from build123d import *

# Parameters (mm, degrees)
SKETCH1_R           = 0.775
BOSS_EXTRUDE1_DEPTH = 18
SKETCH2_R           = 1.5
BOSS_EXTRUDE2_DEPTH = 1
SKETCH3_R           = 2
BOSS_EXTRUDE4_DEPTH = 10
SKETCH5_W           = 0.7
SKETCH5_H           = 0.5
FILLET1_R           = 0.1


with BuildPart() as part:
    # Sketch1 → Boss-Extrude1 (new body)
    with BuildSketch(Plane.XY):
        Circle(SKETCH1_R)
    extrude(amount=BOSS_EXTRUDE1_DEPTH)

    # Sketch2 → Boss-Extrude2 (add)
    with BuildSketch(Plane.XY.offset(18)):
        Circle(SKETCH2_R)
    extrude(amount=BOSS_EXTRUDE2_DEPTH)

    # Sketch3 → Boss-Extrude4 (add)
    with BuildSketch(Plane(origin=(0, 0, 0), x_dir=(-1, 0, 0), z_dir=(0, 0, -1))):
        Circle(SKETCH3_R)
    extrude(amount=BOSS_EXTRUDE4_DEPTH)

    # Sketch5 → Cut-Revolve1 (revolve, cut)
    with BuildSketch(Plane(origin=(0, 0, 0), x_dir=(0, 0, -1), z_dir=(1, 0, 0))):
        with Locations((8.15, 1.75)):
            Rectangle(SKETCH5_W, SKETCH5_H)
    revolve(axis=Axis((0, 0, 0), (0, 0, -1)), mode=Mode.SUBTRACT)

    # Fillet1
    fillet1_edges = [part.edges().sort_by_distance(p)[0] for p in [
        (-1.5, 0, 18),
        (-1.5, 0, 19),
        (2, 0, 0),
        (2, 0, -10),
    ]]
    fillet(fillet1_edges, radius=FILLET1_R)


solid = part.part
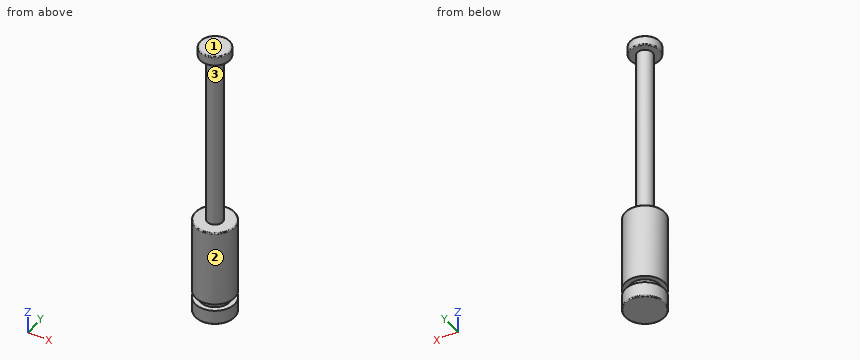
For this review, take the finished solid that the model builds, in its own axes (mm). Face numbers are marked on the shaded views. Round coordinates to 2 decimals unless told otherwise and drop trailing zeros. Loops run counter-clockwise (first coordinate to the right, second up) from the corner with the lowest first, then second, coordinate; pieces in that order, holes last. Notation, with made-up numbers: (-38.5, 50.25) - (4.5, 50.25) arc R12 ccw to (4.5, 57.25) - close; hole circle Ø9 at (20, -21). An arc over 180 degrees is marked (long way). Use one line per item in the form item = value.
1) Clearance check with flat-ended pins moving along their axes: P1, Ø2, axis at x = 1.5, z = 3.5, coming from the +Y side; P2, Ø1.5, axis at y = -0.5, z = 11, coming from the +X side (3 decimals); P3, Ø1, axis at x = 1, y = 1.5, coming from the +Z side. State where each tip first meets the part, or that it passes through.
Solutions:
P1 = 0.59
P2 = 0.775
P3 = 19
2) We need section C-C on z = 17.25. Write out the cut boundary in (x, y) (3 decimals), then the cut area to 3 significant figures.
Solutions:
outline = circle Ø1.55 at (0, 0)
area = 1.89 mm2
3) Wall thickness on probe 1 along Z at (x, y) = (-1.7, 0); probe 2 along Z at (x, y) = (-0.65, 0.65); probe 3 along X at (y, z) = (0.1, 14.75): over which ranges is each line inside the solid? List them lowest first.
Solutions:
probe_1 = -10 to -8.5, -7.8 to 0
probe_2 = -10 to 0, 18 to 19
probe_3 = -0.77 to 0.77
4) Mouldability with a two-part tool opening along Z and no side actions: class the marked faces 1, 2 and 3 as pulls with the +Z half, pulls with the -Z half, needs draft (parallel to the pull), parting line crosses it, or undercut.
Solutions:
face_1 = pulls with the +Z half
face_2 = needs draft
face_3 = undercut
5) We need section A-A on y = 0. Write out the cut boundary in (x, z) (3 decimals).
Solutions:
outline = (-2, -9.9) arc R0.1 ccw to (-1.9, -10) - (1.9, -10) arc R0.1 ccw to (2, -9.9) - (2, -8.5) - (1.5, -8.5) - (1.5, -7.8) - (2, -7.8) - (2, -0.1) arc R0.1 ccw to (1.9, 0) - (0.775, 0) - (0.775, 18) - (1.4, 18) arc R0.1 ccw to (1.5, 18.1) - (1.5, 18.9) arc R0.1 ccw to (1.4, 19) - (-1.4, 19) arc R0.1 ccw to (-1.5, 18.9) - (-1.5, 18.1) arc R0.1 ccw to (-1.4, 18) - (-0.775, 18) - (-0.775, 0) - (-1.9, 0) arc R0.1 ccw to (-2, -0.1) - (-2, -7.8) - (-1.5, -7.8) - (-1.5, -8.5) - (-2, -8.5) - close
